Solid Edge part; units mm, degrees
sketch "Sketch1" plane through (0, 0, 0) normal (0, 0, 1) x (1, 0, 0)
  line L0 (-2.7678, -7.7019) -> (-12.1633, -7.7019)
  line L1 (-12.1633, -7.7019) -> (-12.1633, -3.6)
  line L2 (-2.1633, -3.6) -> (-12.1633, -3.6)
  arc A0 (-2.1633, 3.6) -> (-2.1633, -3.6) centre (0, 0) cw
  line L3 (-2.1633, 3.6) -> (-12.1633, 3.6)
  line L4 (-12.1633, 7.7019) -> (-12.1633, 3.6)
  line L5 (-2.7678, 7.7019) -> (-12.1633, 7.7019)
  arc A1 (-2.7678, 7.7019) -> (-1.7032, 7.8166) centre (-2.7678, 12.7019) ccw
  arc A2 (-1.7032, 7.8166) -> (-1.7032, -7.8166) centre (0, 0) cw
  arc A3 (-2.7678, -7.7019) -> (-1.7032, -7.8166) centre (-2.7678, -12.7019) cw
extrude "Protrusion1" add sketch "Sketch1" along normal blind 12
sketch "Sketch2" plane through (-7.4655, -7.7019, 6) normal (0, -1, 0) x (1, 0, 0)
  circle A0 centre (0, 0) radius 5.5
extrude "Cutout1" cut sketch "Sketch2" along normal through all
sketch "Sketch3" plane through (-7.4655, -7.7019, 6) normal (0, -1, 0) x (1, 0, 0)
  line L0 (0, 3.8868) -> (-1.9422, 1.8756)
  line L1 (1.9422, 1.8756) -> (0, 3.8868)
  arc A0 (1.9422, 1.8756) -> (-1.9422, 1.8755) centre (0, 0) cw
extrude "Cutout2" cut sketch "Sketch3" against normal through all
sketch "Sketch4" plane through (40, 0, 0) normal (1, 0, 0) x (0, 1, 0)
  line L0 (8, 0) -> (8, 12)
  line L1 (4, 12) -> (8, 12)
  line L2 (4, 12) -> (4, 4)
  line L3 (4, 4) -> (-4, 4)
  line L4 (-4, 4) -> (-4, 0)
  line L5 (8, 0) -> (-4, 0)
  dimension "D1" = 8
extrude "ExtrudedProtrusion_2" add sketch "Sketch4" against normal up to next
sketch "Sketch5" plane through (-7.4655, 7.7019, 6) normal (0, 1, 0) x (1, 0, 0)
  circle A0 centre (0, 0) radius 5.5
extrude "Cutout3" cut sketch "Sketch5" along normal through all
fillet "Round_1" radius 4 1 edges at (6.9282, -4, 2)
sketch "Sketch6" plane through (0, 0, 0) normal (0, 0, 1) x (1, 0, 0)
  arc A0 (22.8729, 4) -> (20.8729, 2) centre (22.8729, 2) ccw
  line L0 (28.9771, 4) -> (22.8729, 4)
  arc A1 (30.9771, 2) -> (28.9771, 4) centre (28.9771, 2) ccw
  line L1 (30.9771, 2) -> (30.9771, -5.7679)
  line L2 (20.8729, 2) -> (20.8729, -5.7679)
extrude "Cutout4" cut sketch "Sketch6" along normal through all material side at (21.494, 3.3789, 0)
sketch "Sketch7" plane through (0, 0, 0) normal (0, 0, 1) x (1, 0, 0)
  circle A0 centre (16.425, 0) radius 1.65
  circle A1 centre (35.425, 0) radius 1.65
extrude "Cutout5" cut sketch "Sketch7" along normal through all
sketch "Sketch8" plane through (-12.1633, 5.651, 6) normal (-1, 0, 0) x (0, -1, 0)
  line L0 (2.051, 6) -> (-2.051, 6)
  line L1 (-2.051, 6) -> (-2.051, -6)
  line L2 (2.051, -6) -> (-2.051, -6)
  line L3 (2.051, 6) -> (2.051, -6)
  line L4 (9.251, 6) -> (9.251, -6)
  line L5 (13.3529, -6) -> (9.251, -6)
  line L6 (13.3529, 6) -> (13.3529, -6)
  line L7 (13.3529, 6) -> (9.251, 6)
extrude "ExtrudedProtrusion_3" add sketch "Sketch8" along normal blind 2
properties material "ABS Plastic, medium impact"
Here's how the part is built. I have some questions about the finished solid (model axes, mm). A direction names the side the tool comes from. Give positions to 0.01 mm unless a question says otherwise; leave off trailing zeros. Order: outer loops, then holes, each group sorted by start corner. A loop starts at its lowest first (then second) coordinate and runs counter-clockwise, first axis right, second up. Notation, with made-up numbers: M -16.5,39.25 L 35.5,39.25 A36 cw 35.5,76.25 Z; hole C -11.5,-26.5 d7. An arc over 180 degrees is marked long. Use a Markdown table: item, result. Add a question column.
1. On a 3-axis mill with a long thin cutter (end or side, diameter ignored), from which of +Z, -Z, +X, -X, +Y, -Y can I reach the whole of each face in a straight line? I mean faces 1 (the cylindrical face through (30.376, 3.43, 1.972)), 2 (the flat face through (37, 1, 4)), 3 (the flat face through (-13, 7.702, 6)), 4 (the flat face through (-6.481, -5.68, 8.867)). Say none if no direction works.
2. If we mould it in two halves opening along X, with no side actions, what happens to faces 5 (the flat face through (-14.163, 6, 6)), 6 (the flat face through (15, -4, 2)), 7 (the cylindrical face through (21.443, 3.399, 1.972)), 8 (the cylindrical face through (36.95, 0.63, 1.97))? For each: +X half, -X half, draft (parallel to the pull), parting line (faces both ways), or undercut.
3. Suppose I cut it at A-A (y = 0). List the corners of the cut face in (x, z) for me (3 decimals), and give its area (3 significant figures).
4. Suppose I cut it at D-D (x = 19). List the corners of the cut face in (y, z) for me.
5. Suppose I cut it at B-B (z = 6). Give the number of separate pieces and of enclosed holes in the cut face, and give its area (3 significant figures).
6. For pin 1 Ø4 at (x, y) = (32.5, 1) entering from +Z; pin 2 Ø5 at (x, z) = (9, 4.5) entering from -Y; pin 3 Ø3 at (x, z) = (-6, 4) entering from -Y, each with a flat end and sliding along its axis, tell me the tip position at first contact or that it passes through.
7. Suppose I cut it at C-C (y = 6). List the corners of the cut face in (x, z) for me, and give its area (3 significant figures).
8. I need wall thicknesses on probe 1 along X at (y, z) = (0, 2.1) (3 decimals); probe 2 along Y at (x, z) = (-4.5, 8.25); probe 3 along Y at (x, z) = (20, 4.75). Which ranges of each line are inside material? Lowest first, please. Write a range as from..to.
Results list:
| question | item | result |
|---|---|---|
| 1 | face 1 | +Z, -Z, -Y |
| 1 | face 2 | +Z, +X, -Y |
| 1 | face 3 | +Z, -Z, -X, +Y |
| 1 | face 4 | +Y, -Y |
| 2 | face 5 | -X half |
| 2 | face 6 | draft |
| 2 | face 7 | undercut |
| 2 | face 8 | undercut |
| 3 | outline | M 4.2,0 L 14.775,0 L 14.775,4 L 8,4 L 8,12 L 4.2,12 Z; M 18.075,0 L 20.873,0 L 20.873,4 L 18.075,4 Z; M 30.977,0 L 33.775,0 L 33.775,4 L 30.977,4 Z; M 37.075,0 L 40,0 L 40,4 L 37.075,4 Z |
| 3 | area | 107 mm² |
| 4 | outline | M -4,0 L 8,0 L 8,12 L 4,12 L 4,4 L -4,4 Z |
| 5 | separate pieces | 3 |
| 5 | enclosed holes | 0 |
| 5 | area | 284 mm² |
| 6 | pin 1 | stops at z = 4 |
| 6 | pin 2 | stops at y = -4.8 |
| 6 | pin 3 | stops at y = -7.7 |
| 7 | outline | M -14.16,0 L 40,0 L 40,12 L -14.16,12 Z; hole M -9.41,7.88 A2.7 ccw long -5.52,7.88 L -7.47,9.89 Z |
| 7 | area | 625 mm² |
| 8 | probe 1 | x = 4.2..14.775, 18.075..20.873, 30.977..33.775, 37.075..40 |
| 8 | probe 2 | y = -7.7..-3.6, 3.6..7.7 |
| 8 | probe 3 | y = 4..8 |
